Autodesk Fusion 360 part; units mm, degrees
sketch "Sketch7" plane through (0, 0, 0) normal (1, 0, 0) x (0, 0, -1)
  line L0 (-40, 0) -> (40, 0)
  line L1 (40, 0) -> (40, 40)
  line L2 (40, 40) -> (65, 40)
  line L3 (65, 40) -> (65, -10)
  line L4 (-40, 0) -> (-40, -10)
  line L5 (0, 0) -> (0, -30) construction
  circle A0 centre (0, -30) radius 9.025
  line L6 (-40, -10) -> (-32.5, -50)
  line L7 (-32.5, -50) -> (32.5, -50)
  line L8 (32.5, -50) -> (65, -10)
  dimension "d98" = 80
  dimension "d99" = 40
  dimension "d100" = 25
  dimension "d101" = 50
  dimension "d102" = 10
  dimension "d103" = 30
  dimension "d104" = 18.05
  dimension "d105" = 7.5
  dimension "d106" = 7.5
  dimension "d107" = 50
extrude "Extrude12" add sketch "Sketch7" along normal blind 40 makes body 1
sketch "Sketch8" plane through (0, 0, 0) normal (0, 1, 0) x (-1, 0, 0)
  line L0 (0, -40) -> (0, 40)
  line L1 (0, 40) -> (-40, 40)
  line L2 (-40, 40) -> (-40, -40)
  line L3 (-40, -40) -> (0, -40)
  line L4 (-40, 20) -> (0, 20) construction
  line L5 (0, -20) -> (-40, -20) construction
  circle A0 centre (-20, 20) radius 10.5
  circle A1 centre (-20, 20) radius 4.25
  circle A2 centre (-20, -20) radius 10.5
  circle A3 centre (-20, -20) radius 4.25
  dimension "d110" = 20
  dimension "d111" = 20
  dimension "d112" = 21
  dimension "d113" = 8.5
extrude "Extrude13" cut sketch "Sketch8" against normal blind 65 contours A0 | A1 | A2 | A3 bodies 1
extrude "Extrude14" add sketch "Sketch8" against normal blind 48 contours A0 | A2 bodies 1
sketch "Sketch9" plane through (0, 0, -40) normal (0, 0, 1) x (1, 0, 0)
  line L0 (0, 40) -> (0, 0)
  line L1 (0, 0) -> (40, 0)
  line L2 (40, 0) -> (40, 40)
  line L3 (40, 40) -> (0, 40)
  line L4 (0, 40) -> (40, 0) construction
  circle A0 centre (20, 20) radius 10.5
  circle A1 centre (20, 20) radius 4.25
  dimension "d118" = 21
  dimension "d119" = 8.5
extrude "Extrude15" cut sketch "Sketch9" against normal blind 25 contours A0 | A1 bodies 1
extrude "Extrude16" add sketch "Sketch9" against normal blind 20 contours A0 bodies 1
fillet "Fillet6" radius 7.5 1 edges at (20, -50, 32.5) on bodies 1
fillet "Fillet6" radius 92.5 1 edges at (20, -10, 40) on bodies 1
fillet "Fillet6" radius 12.5 1 edges at (20, -50, -32.5) on bodies 1
fillet "Fillet6" radius 32.5 1 edges at (20, -10, -65) on bodies 1
fillet "Fillet6" radius 10 2 edges at (40, 40, -52.5) (0, 40, -52.5) on bodies 1
chamfer "Chamfer2" distance 2 distance2 2 26 edges at (40, 15.7694, -65) (37.0711, 37.0711, -65) (20, 40, -65) (2.9289, 37.0711, -65) (0, 15.7694, -65) (0, -9.335, -63.127) (0, -32.1689, -46.9877) (0, -48.7867, -31.9225) (0, -50, -0.1374) (0, -48.2713, 31.0653) (0, -31.1659, 36.0314) (0, -9.9631, 39.6031) (0, -0.7015, 40) (40, -0.7015, 40) (40, -9.9631, 39.6031) (40, -31.1659, 36.0314) (40, -48.2713, 31.0653) (40, -50, -0.1374) (40, -48.7867, -31.9225) (40, -32.1689, -46.9877) (40, -9.335, -63.127) (37.0711, 37.0711, -40) (40, 15, -40) (0, 15, -40) (2.9289, 37.0711, -40) (20, 40, -40) measured on face at (40, -24.2407, -28.2919) measured on face at (30.4758, 39.9887, -48.3333) measured on face at (36.7942, 16.658, -65) measured on face at (9.5242, 39.9887, -48.3333) measured on face at (0, -24.2407, -28.2919) measured on face at (13.3333, -4.342, -64.4635) measured on face at (21.3822, -27.9314, -50.4307) measured on face at (3.9312, -49.9391, -27.7824) measured on face at (36.4044, -50, -5.0795) measured on face at (7.7211, -44.5562, 33.4882) measured on face at (21.8485, -27.0997, 36.7938) measured on face at (13.3333, -10.911, 39.51) measured on face at (26.6667, -0.4677, 40) measured on face at (40, -24.2407, -28.2919) measured on face at (13.3333, -10.911, 39.51) measured on face at (40, -24.2407, -28.2919) measured on face at (32.2789, -49.9654, 26.9948) measured on face at (40, -24.2407, -28.2919) measured on face at (32.1375, -47.1192, -34.5329) measured on face at (40, -24.2407, -28.2919) measured on face at (13.3333, -4.342, -64.4635) measured on face at (30.4758, 39.9887, -48.3333) measured on face at (40, -24.2407, -28.2919) measured on face at (0, -24.2407, -28.2919) measured on face at (9.5242, 39.9887, -48.3333) measured on face at (16.6667, 40, -48.3333) on bodies 1
chamfer "Chamfer2" distance 0.6 distance2 0.6 3 faces at (24.2447, 19.7882, -53.3333) (15.7553, -32, -20.2118) (15.7553, -32, 19.7882) on bodies 1
chamfer "Chamfer2" distance 0.6 distance2 2 1 edges at (40, -26.7364, 8.4143) measured on face at (40, -24.2407, -28.2919) on bodies 1
chamfer "Chamfer2" distance 2 distance2 0.6 1 edges at (0, -26.7364, 8.4143) measured on face at (26.6667, -30.4499, -9.0138) on bodies 1
copy_body "Body->Comp2" bodies 1 removing the originals makes body 2 in component "wheel stand hinge point"
component "wheel stand hinge point" placed x (1, 0, 0) y (0, 1, 0) z (0, 0, 1) at (0, 0, 0)
Source: CAD feature listing. Evaluate the final solid. Frame: model axes, mm. A direction names the side the tool comes from. Give positions to 0.01 mm unless a question says otherwise; leave off trailing zeros. Write each loop counter-clockwise with the first axis right and the second up, starting at its lowest first coordinate (ties: lowest second). Pieces come first, ordered by that corner, then holes. Notation, with made-up numbers: M 4,11 L 48,11 A33 ccw 48,39 Z; hole C 50.5,27.25 d8. An arc over 180 degrees is marked long. Return JSON: item names as keys, results as strings. Group by question number.
1) Ray query, L1, parallel to Z at x = 10, y = 13; L2, parallel to Z at x = 20, y = -49.15; L3, parallel to Z at x = 20, y = -22. Return the intervals inside material, ascending.
2) First-contact query: pin 1 Ø20 at (x, z) = (16.5, -21.5) entering from +Y; pin 2 Ø6.5 at (x, z) = (23, -24) entering from -Y; pin 3 Ø17 at (x, y) = (19.5, 20) entering from -Z. Flat tips, straight axial feed; report the tip coordinate or a pass-through.
3) Cut plane C-C, the plane x = 20. Give the number of separate pieces and of enclosed holes in the cut face, then the cut area to 3 significant figures.
4) Set-up query: faces 5 (the face through (20, -50, 0)), 6 (the face through (21.37, -48.99, 30.41)), 7 (the face through (33.276, -48.225, 31.121)). Return all of +Z, -Z, +X, -X, +Y, -Y with unobstructed straight access to the full face (end or side cutting, diameter ignored); none if empty.
5) Cut plane A-A, the plane z = 20. Output: boundary loops of the cut face in (x, y), then the cut area to 3 significant figures.
6) Cut plane D-D, the plane y = -30. Output: boundary loops of the cut face in (x, z) (3 decimals), then the cut area to 3 significant figures.
7) Draft query along Z for faces 1 (the face through (39.208, -47.38, 30.247)), 2 (the face through (39.208, -47.665, -31.467)), 3 (the face through (2.85, 36.99, -52.65)), 4 (the face through (18, -48, -25)). Return one class per face: released by +Z, released by -Z, zero draft, split by the parting line, or undercut.
8) Cut plane B-B, the plane y = 20. Output: boundary loops of the cut face in (x, z).
Data:
{
 "1": {"L1": "z = -65 to -40", "L2": "z = -32.21 to -30.5, -9.5 to 9.5, 30.5 to 31.45", "L3": "z = -55.25 to -24.25, -15.75 to -4.18, 4.18 to 15.75, 24.25 to 37.75"},
 "2": {"pin 1": "stops at y = 0", "pin 2": "stops at y = -48", "pin 3": "stops at z = -60"},
 "3": {"separate pieces": "4", "enclosed holes": "1", "area": "3,990 mm²"},
 "4": {"face 5": "+Z, -Z, +X, -X, -Y", "face 6": "-Y", "face 7": "+Z, +X, -Y"},
 "5": {"outline": "M 0,-48 L 2,-50 L 9.5,-50 L 9.5,-48 L 15.15,-48 L 15.75,-47.4 L 15.75,-0.6 L 15.15,0 L 0,0 Z; M 24.25,-47.4 L 24.85,-48 L 30.5,-48 L 30.5,-50 L 38,-50 L 40,-48 L 40,0 L 24.85,0 L 24.25,-0.6 Z", "area": "1,550 mm²"},
 "6": {"outline": "M 0,-46.173 L 2,-48.75 L 38,-48.75 L 40,-46.173 L 40,-9.625 L 38,-9.025 L 2,-9.025 L 0,-9.625 Z; M 0,9.625 L 2,9.025 L 38,9.025 L 40,9.625 L 40,34.215 L 38,36.25 L 2,36.25 L 0,34.215 Z; hole C 20,-20 d8.5; hole C 20,20 d8.5", "area": "2,550 mm²"},
 "7": {"face 1": "released by +Z", "face 2": "released by -Z", "face 3": "zero draft", "face 4": "undercut"},
 "8": {"outline": "M 0,-63 L 2,-65 L 9.5,-65 L 9.5,-60 L 15.15,-60 L 15.75,-59.4 L 15.75,-40.6 L 15.15,-40 L 2,-40 L 0,-42 Z; M 24.25,-59.4 L 24.85,-60 L 30.5,-60 L 30.5,-65 L 38,-65 L 40,-63 L 40,-42 L 38,-40 L 24.85,-40 L 24.25,-40.6 Z"}
}
